For this review, use the dimensioned drawing (mm, ordinates from the lowest corner) and the shaded views. A direction names the side the tool comes from. Coordinates: 2 decimals unless noted, no trailing zeros. Order: outer loops, then holes, each group sorted by start corner. A loop starts at its lowest first (then second) coordinate and runs counter-clockwise, first axis right, second up. Notation, with made-up numbers: M 35.5,49.25 L 68.5,49.25 A29 ccw 68.5,85.25 Z; hole C 0.25,68 d3. An arc over 180 degrees is marked long. Answer in a Markdown table with one row per item.
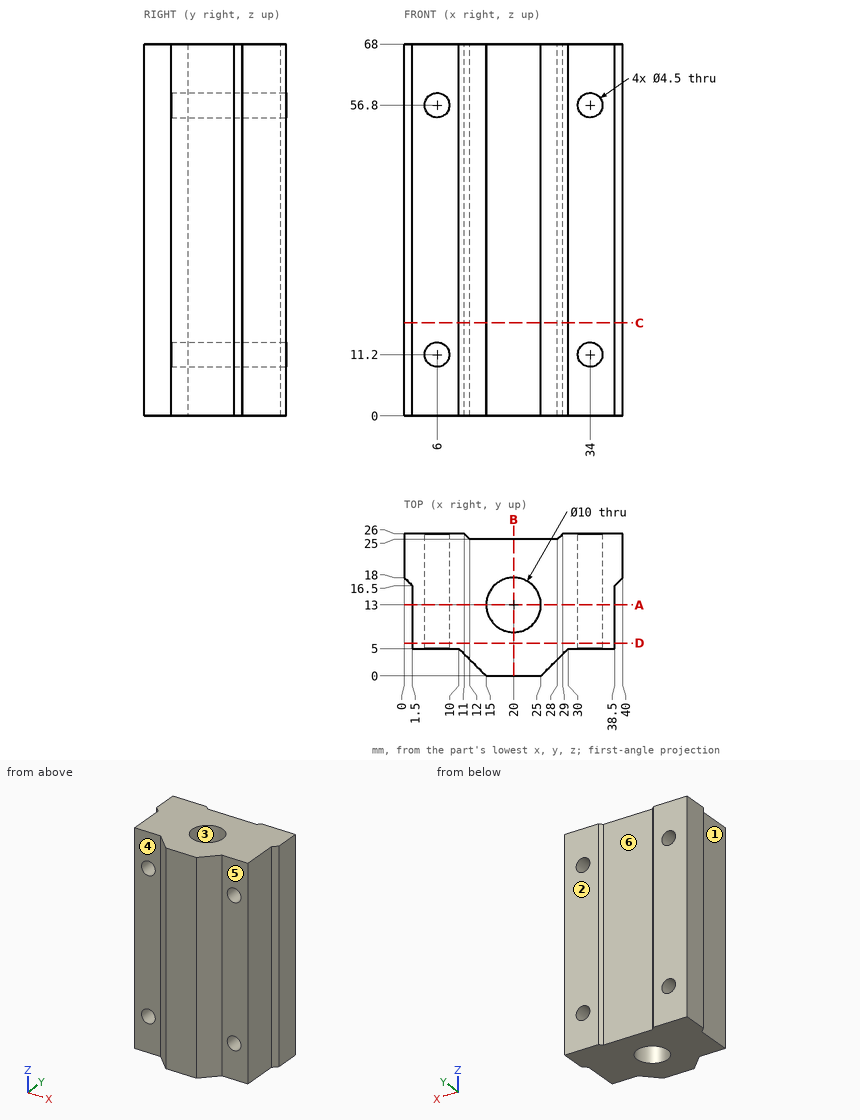
(1) Insertion check: pin 1 Ø10 at (x, z) = (31, 29) entering from -Y; pin 2 Ø6 at (x, z) = (34, 11.2) entering from -Y; pin 3 Ø3.5 at (y, z) = (11.5, 33) entering from -X. Each pin has a flat end and moves straight along its axis. Give the tip position at first contact, or say it passes through.
Return value:
| item | result |
|---|---|
| pin 1 | stops at y = 1 |
| pin 2 | stops at y = 5 |
| pin 3 | stops at x = 1.5 |
(2) Add section B-B, the plane x = 20. Give the boundary of the cut face in (y, z), and give its area (3 significant figures).
Return value:
| item | result |
|---|---|
| outline | M 0,0 L 8,0 L 8,68 L 0,68 Z; M 18,0 L 25,0 L 25,68 L 18,68 Z |
| area | 1,020 mm2 |
(3) Add section D-D, the plane y = 6. Give the boundary of the cut face in (x, z), and give its area (3 significant figures).
Return value:
| item | result |
|---|---|
| outline | M 1.5,0 L 38.5,0 L 38.5,68 L 1.5,68 Z; hole C 6,11.2 d4.5; hole C 6,56.8 d4.5; hole C 34,11.2 d4.5; hole C 34,56.8 d4.5 |
| area | 2,450 mm2 |
(4) Add section A-A, the plane y = 13. Give the boundary of the cut face in (x, z).
Return value:
| item | result |
|---|---|
| outline | M 1.5,0 L 15,0 L 15,68 L 1.5,68 Z; M 25,0 L 38.5,0 L 38.5,68 L 25,68 Z; hole C 6,11.2 d4.5; hole C 6,56.8 d4.5; hole C 34,11.2 d4.5; hole C 34,56.8 d4.5 |
(5) Draft analysis for pull direction X (two halves, no side actions). For the marked faces 1, 2 and 3, state which applies: pulls with the +X half, pulls with the -X half, needs draft (parallel to the pull), parting line crosses it, or undercut.
Return value:
| item | result |
|---|---|
| face 1 | pulls with the -X half |
| face 2 | needs draft |
| face 3 | undercut |
(6) For line 1 along X through (y, z) = (20.5, 56.8); line 2 along Z through (x, y) = (6, 13.25); line 3 along X through (y, z) = (12, 11.2), list the stretches that pass through material, from the lowest coordinate up. Write a range as from..to.
Return value:
| item | result |
|---|---|
| line 1 | x = 0..3.75, 8.25..31.75, 36.25..40 |
| line 2 | z = 0..8.95, 13.45..54.55, 59.05..68 |
| line 3 | x = 1.5..3.75, 8.25..15.1, 24.9..31.75, 36.25..38.5 |
(7) Add section C-C, the plane z = 17. Give the boundary of the cut face in (x, y), and give its area (3 significant figures).
Return value:
| item | result |
|---|---|
| outline | M 0,18 L 1.5,16.5 L 1.5,5 L 10,5 L 15,0 L 25,0 L 30,5 L 38.5,5 L 38.5,16.5 L 40,18 L 40,26 L 29,26 L 28,25 L 12,25 L 11,26 L 0,26 Z; hole C 20,13 d10 |
| area | 783 mm2 |
(8) For the marked faces 4, 5 and 6, list the 3-axis set-ups (+Z, -Z, +X, -X, +Y, -Y) from which the entire face can be reached by the end or side of a thin tool; tool diameter is ignored.
Return value:
| item | result |
|---|---|
| face 4 | +Z, -Z, -X, -Y |
| face 5 | +Z, -Z, +X, -Y |
| face 6 | +Z, -Z, +Y |
